from build123d import *

# Parameters (mm, degrees)
F0_R     = 50.8
F1_DEPTH = 25.4
F2_R     = 12.7
F3_R     = 12.69999
F5_D     = 2.999994


# Not quite as in the source:
# - a fillet or chamfer is up to 0.001 mm smaller than in the source, because OpenCascade refuses the exact size


with BuildPart() as f1:
    # F0 (on Right) → F1 (new body)
    with BuildSketch(Plane.YZ):
        Circle(F0_R)
    extrude(amount=F1_DEPTH)

    # F2
    f2_edges = [f1.edges().sort_by_distance(p)[0] for p in [
        (25.4, -50.8, 0),
    ]]
    fillet(f2_edges, radius=F2_R)

    # F3 (radius 12.7 in the source; OpenCascade refuses exactly that, so slightly less here)
    f3_edges = [f1.edges().sort_by_distance(p)[0] for p in [
        (0, -50.8, 0),
    ]]
    fillet(f3_edges, radius=F3_R)

    # F5 (through all)
    with Locations(Plane.YZ.offset(25.4)):
        with Locations((0, 0)):
            Hole(F5_D / 2)


solid = f1.part
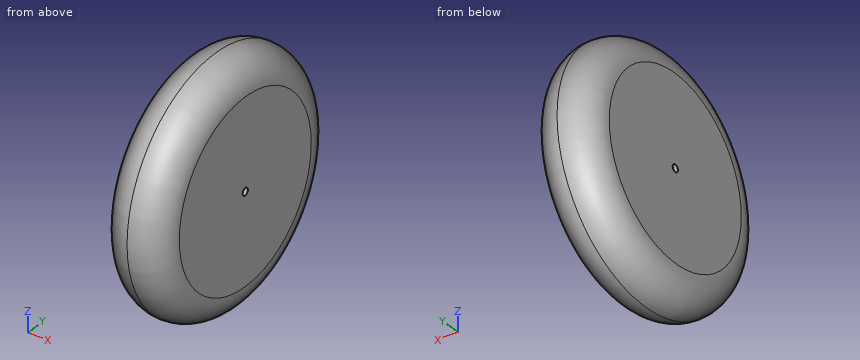
The listing builds one solid part. Answer for the finished solid, in the listing's coordinates (mm). Give positions to 0.01 mm unless a question says otherwise; leave off trailing zeros. Loops run counter-clockwise (first coordinate to the right, second up) from the corner with the lowest first, then second, coordinate; pieces in that order, holes last.
Item 1: Each of these flat-tipped pins is pushed along its axis until it touches: pin 1 Ø10 at (x, z) = (20, -6.5) entering from -Y; pin 2 Ø6 at (x, y) = (12, 37.5) entering from -Z; pin 3 Ø10 at (x, y) = (7.5, 27.5) entering from -Z; pin 4 Ø2.5 at (y, z) = (0, 0) entering from -X. Where does it stop, or does it pass through?
Derived:
pin 1: stops at y = -50.31
pin 2: stops at z = -37.27
pin 3: stops at z = -44.89
pin 4: passes through
Item 2: Find the intervals of material crossed by line 1 along Z through (x, y) = (12.75, 0); line 2 along Z through (x, y) = (7.25, 0); line 3 along X through (y, z) = (44.5, -19), in increasing order.
Derived:
line 1: z = -50.8 to -1.5, 1.5 to 50.8
line 2: z = -49.57 to -1.5, 1.5 to 49.57
line 3: x = 5.25 to 20.15
Item 3: A cutting plane is placed at C-C (x = 18.5). Give the vertices of the cut face in (y, z).
Derived:
outline: circle Ø98.8 at (0, 0); hole circle Ø3 at (0, 0)
